from build123d import *

# Parameters (mm, degrees)
SKETCH2_W           = 115
SKETCH2_H           = 120
SKETCH2_R           = 2.25
BOSS_EXTRUDE1_DEPTH = 5
SKETCH3_R           = 5
BOSS_EXTRUDE2_DEPTH = 20
SKETCH6_W           = 2.5
SKETCH6_H           = 18
SKETCH8_W           = 18
SKETCH8_H           = 2.5
SKETCH9_W           = 18
SKETCH9_H           = 2.5
FILLET1_R           = 10


with BuildPart() as part:
    # Sketch2 → Boss-Extrude1 (new body)
    with BuildSketch(Plane.XY):
        Rectangle(SKETCH2_W, SKETCH2_H)
        with Locations((50, 52.5)):
            Circle(SKETCH2_R, mode=Mode.SUBTRACT)
        with Locations((50, -52.5)):
            Circle(SKETCH2_R, mode=Mode.SUBTRACT)
        with Locations((-50, -52.5)):
            Circle(SKETCH2_R, mode=Mode.SUBTRACT)
        with Locations((-50, 52.5)):
            Circle(SKETCH2_R, mode=Mode.SUBTRACT)
    extrude(amount=-BOSS_EXTRUDE1_DEPTH)

    # Sketch3 → Boss-Extrude2 (add)
    with BuildSketch(Plane.XY):
        Circle(SKETCH3_R)
    extrude(amount=BOSS_EXTRUDE2_DEPTH)

    # Sketch4 → Revolve3 (revolve)
    with BuildSketch(Plane(origin=(0, 0, 0), x_dir=(1, 0, 0), z_dir=(0, 1, 0))):
        with BuildLine():
            Line((0, -12.5), (0, -27.5))
            ThreePointArc((0, -27.5), (7.5, -20), (0, -12.5))
        make_face()
    revolve(axis=Axis((0, 0, -22.886774461), (0, 0, 1)))

    # Sketch6 → Cut-Revolve1 (revolve, cut)
    with BuildSketch(Plane(origin=(0, 0, 0), x_dir=(0, 0, -1), z_dir=(1, 0, 0))):
        with Locations((-18.75, 6)):
            Rectangle(SKETCH6_W, SKETCH6_H)
    revolve(axis=Axis((0, 42.177542576, 20), (0, -1, 0)), mode=Mode.SUBTRACT)

    # Sketch8 → Cut-Revolve2 (revolve, cut)
    with BuildSketch(Plane(origin=(0, 0, 0), x_dir=(0, 0, -1), z_dir=(1, 0, 0))):
        with Locations((-26, 1.25)):
            Rectangle(SKETCH8_W, SKETCH8_H)
    revolve(axis=Axis((0, 0, 46.4260406), (0, 0, -1)), mode=Mode.SUBTRACT)

    # Sketch9 → Cut-Revolve3 (revolve, cut)
    with BuildSketch(Plane(origin=(0, 0, 0), x_dir=(1, 0, 0), z_dir=(0, 1, 0))):
        with Locations((6, -18.75)):
            Rectangle(SKETCH9_W, SKETCH9_H)
    revolve(axis=Axis((-16.030191757, 0, 20), (1, 0, 0)), mode=Mode.SUBTRACT)

    # Fillet1
    fillet1_edges = [part.edges().sort_by_distance(p)[0] for p in [
        (-57.5, 60, -2.5),
        (57.5, 60, -2.5),
        (57.5, -60, -2.5),
        (-57.5, -60, -2.5),
    ]]
    fillet(fillet1_edges, radius=FILLET1_R)


solid = part.part
For this review, take the finished solid that the model builds, in its own axes (mm). A direction names the side the tool comes from. Round coordinates to 2 decimals unless told otherwise and drop trailing zeros. Order: outer loops, then holes, each group sorted by start corner. A loop starts at its lowest first (then second) coordinate and runs counter-clockwise, first axis right, second up. Notation, with made-up numbers: (49, 4) -> (106, 4) arc R26 cw to (106, 36) -> close; hole circle Ø6 at (6.25, 72.5). An arc over 180 degrees is marked (long way). Write item = value, one per line. Start each with the question number.
1) To check wall thickness, follow line 1 (Y direction, x = -50, z = -2.9); line 2 (X direction, y = -52, z = -3); line 3 (Z direction, x = -17, y = -19.5). State the ranges of each line that lie inside material, in increasing order. Write a range as from..to.
2) Take a section at D-D on x = -50. State the section outline as (y, z) points, plus the area to 3 significant figures.
3) Take a section at B-B on y = 0. State the section outline as (x, z) points, plus the area to 3 significant figures.
4) Insertion check: pin 1 (4 mm diameter, centred on y = 1, z = 21, fed in from +X); pin 2 (4 mm diameter, centred on x = -50, y = -52.5, fed in from +Z); pin 3 (8 mm diameter, centred on y = 0, z = 20, fed in from -X); pin 4 (3 mm diameter, centred on x = 0, z = 20, fed in from +Y). Each pin has a flat end and moves straight along its axis. Give the tip position at first contact, or say it passes through.
5) Take a section at A-A on x = 0. State the section outline as (y, z) points.
6) Take a section at C-C on y = 52.5. State the section outline as (x, z) points, plus the area to 3 significant figures.
7) The part is to be moulded in two halves that separate along Z. For faces 1 (the face through (4.5, 0.1, 22.5)), 2 (the face through (0, 0, 17)), 3 (the face through (-1.08, -4.88, 7.1)), 4 (the face through (-51.66, 54.02, -2.46)), say which applies: +Z half, -Z half, draft (parallel to the pull), parting line (faces both ways), or undercut.
8) Tool access review of faces 5 (the face through (-2.649, 0.11, 22.498)), 6 (the face through (0.11, -2.649, 22.498)), 7 (the face through (0.1, -2.5, 24.4)): name each direction out of +Z, -Z, +X, -X, +Y, -Y from which nothing blocks a thin tool from reaching the whole face with its end or side.
Verdict:
q1.line_1 = -59.68..-54.75, -50.25..50.25, 54.75..59.68
q1.line_2 = -57.3..-52.19, -47.81..47.81, 52.19..57.3
q1.line_3 = -5..0
q2.outline = (-59.68, -5) -> (-54.75, -5) -> (-54.75, 0) -> (-59.68, 0) -> close; (-50.25, -5) -> (50.25, -5) -> (50.25, 0) -> (-50.25, 0) -> close; (54.75, -5) -> (59.68, -5) -> (59.68, 0) -> (54.75, 0) -> close
q2.area = 552 mm2
q3.outline = (-57.5, -5) -> (57.5, -5) -> (57.5, 0) -> (5, 0) -> (5, 14.41) arc R7.5 ccw to (7.07, 17.5) -> (2.5, 17.5) -> (2.5, 17) -> (-2.5, 17) -> (-2.5, 17.5) -> (-3, 17.5) -> (-3, 22.5) -> (-2.5, 22.5) -> (-2.5, 27.07) arc R7.5 ccw to (-5, 14.41) -> (-5, 0) -> (-57.5, 0) -> close; (2.5, 22.5) -> (7.07, 22.5) arc R7.5 ccw to (2.5, 27.07) -> close
q3.area = 804 mm2
q4.pin_1 = 7.07
q4.pin_2 = through
q4.pin_3 = -7.5
q4.pin_4 = -3
q5.outline = (-60, -5) -> (60, -5) -> (60, 0) -> (5, 0) -> (5, 14.41) arc R7.5 ccw to (7.07, 17.5) -> (2.5, 17.5) -> (2.5, 17) -> (-2.5, 17) -> (-2.5, 17.5) -> (-3, 17.5) -> (-3, 22.5) -> (-2.5, 22.5) -> (-2.5, 27.07) arc R7.5 ccw to (-5, 14.41) -> (-5, 0) -> (-60, 0) -> close; (2.5, 22.5) -> (7.07, 22.5) arc R7.5 ccw to (2.5, 27.07) -> close
q6.outline = (-57.18, -5) -> (-52.25, -5) -> (-52.25, 0) -> (-57.18, 0) -> close; (-47.75, -5) -> (47.75, -5) -> (47.75, 0) -> (-47.75, 0) -> close; (52.25, -5) -> (57.18, -5) -> (57.18, 0) -> (52.25, 0) -> close
q6.area = 527 mm2
q7.face_1 = undercut
q7.face_2 = +Z half
q7.face_3 = undercut
q7.face_4 = draft
q8.face_5 = +X
q8.face_6 = +Y
q8.face_7 = +Z
